For this review, take the finished solid that the model builds, in its own axes (mm). A direction names the side the tool comes from. Round coordinates to 2 decimals unless told otherwise and drop trailing zeros. Write each loop counter-clockwise with the first axis right and the second up, starting at its lowest first coordinate (ties: lowest second). Pieces come first, ordered by that corner, then holes. Notation, with made-up numbers: (42.5, 15.25) -> (51.5, 15.25) arc R25 ccw to (51.5, 35.25) -> close; hole circle Ø11 at (57, -23). An arc over 180 degrees is marked (long way). Answer in a Markdown table with one row per item. Add a question column.
Solid Edge part; units mm, degrees
sketch "Sketch1" plane through (0, 0, 0) normal (0, 0, 1) x (1, 0, 0)
  line L0 (-28.9647, 0) -> (-28.9647, 39.8)
  line L1 (-28.9647, 39.8) -> (-11.9647, 39.8)
  arc A0 (-11.9647, 39.8) -> (-8.8647, 38.9694) centre (-11.9647, 33.6) cw
  line L2 (14.8644, 25.2694) -> (-8.8647, 38.9694)
  arc A1 (14.8644, 14.5306) -> (14.8644, 25.2694) centre (11.7644, 19.9) ccw
  line L3 (-8.8647, 0.8306) -> (14.8644, 14.5306)
  arc A2 (-11.9647, 0) -> (-8.8647, 0.8306) centre (-11.9647, 6.2) ccw
  line L4 (-28.9647, 0) -> (-11.9647, 0)
extrude "Protrusion1" add sketch "Sketch1" along normal blind 10
sketch "Sketch2" plane through (-5.5002, 19.9, 10) normal (0, 0, 1) x (1, 0, 0)
  circle A0 centre (1.4355, 0.0168) radius 2.65
extrude "ExtrudedCutout_1" cut sketch "Sketch2" against normal blind 233.7228
sketch "Sketch3" plane through (-5.5002, 19.9, 0) normal (0, 0, -1) x (1, 0, 0)
  line L0 (-3.6741, -2.9668) -> (-3.6741, 2.9332)
  line L1 (-3.6741, 2.9332) -> (1.4355, 5.8832)
  line L2 (1.4355, 5.8832) -> (6.545, 2.9332)
  line L3 (6.545, 2.9332) -> (6.545, -2.9668)
  line L4 (6.545, -2.9668) -> (1.4355, -5.9168)
  line L5 (1.4355, -5.9168) -> (-3.6741, -2.9668)
extrude "ExtrudedCutout_2" cut sketch "Sketch3" against normal blind 4.9
1. The part is to be moulded in two halves that separate along X. For faces 1 (the flat face through (1.045, 20, 2)), 2 (the flat face through (-9.174, 20, 2)), 3 (the cylindrical face through (17.964, 19.991, 4.93)), 4 (the flat face through (-10, 20, 0)), say which applies: pulls with the +X half, pulls with the -X half, needs draft (parallel to the pull), parting line crosses it, or undercut.
2. For L1, parallel to Z at x = -5.5, y = 15; L2, parallel to X at y = 19, z = 9.75; L3, parallel to Y at x = -6.5, z = 5, list the stretches that pass through material, from the lowest coordinate up. Write a range as [from, to].
3. We need section D-D (y = 16). Write out the cut boundary in (x, z), plus the area to 3 significant figures.
4. Tool access review of faces 5 (the flat face through (-28.965, 20, 5)), 6 (the flat face through (-6.655, 15.512, 2.416)): name each direction out of +Z, -Z, +X, -X, +Y, -Y from which nothing blocks a thin tool from reaching the whole face with its end or side.
5. We need section A-A (y = 21). Write out the cut boundary in (x, z), plus the area to 3 significant figures.
6. We need section C-C (x = -0.5). Write out the cut boundary in (y, z), plus the area to 3 significant figures.
7. We need section B-B (z = 2.5). Write out the cut boundary in (x, y), plus the area to 3 significant figures.
8. Clearance check with flat-ended pins moving along their axes: pin 1 Ø2 at (y, z) = (27, 2.5) entering from +X; pin 2 Ø4 at (y, z) = (19.5, 3.5) entering from +X; pin 3 Ø1.5 at (y, z) = (4, 6.5) entering from +X; pin 4 Ø2 at (x, z) = (-2, 6.5) entering from +Y. State where each tip first meets the part, or that it passes through.
Response:
| question | item | result |
|---|---|---|
| 1 | face 1 | undercut |
| 1 | face 2 | undercut |
| 1 | face 3 | pulls with the +X half |
| 1 | face 4 | needs draft |
| 2 | L1 | [4.9, 10] |
| 2 | L2 | [-28.96, -6.55], [-1.58, 17.9] |
| 2 | L3 | [2.2, 18.87], [20.96, 37.6] |
| 3 | outline | (-28.96, 0) -> (-7.5, 0) -> (-7.5, 4.9) -> (-0.63, 4.9) -> (-0.63, 0) -> (16.58, 0) -> (16.58, 10) -> (-28.96, 10) -> close |
| 3 | area | 422 mm2 |
| 4 | face 5 | +Z, -Z, -X, +Y, -Y |
| 4 | face 6 | -Z |
| 5 | outline | (-28.96, 0) -> (-9.17, 0) -> (-9.17, 4.9) -> (-6.48, 4.9) -> (-6.48, 10) -> (-28.96, 10) -> close; (-1.65, 4.9) -> (1.04, 4.9) -> (1.04, 0) -> (17.87, 0) -> (17.87, 10) -> (-1.65, 10) -> close |
| 5 | area | 394 mm2 |
| 6 | outline | (5.66, 0) -> (16.07, 0) -> (16.07, 4.9) -> (23.76, 4.9) -> (23.76, 0) -> (34.14, 0) -> (34.14, 10) -> (5.66, 10) -> close |
| 6 | area | 247 mm2 |
| 7 | outline | (-28.96, 0) -> (-11.96, 0) arc R6.2 ccw to (-8.86, 0.83) -> (14.86, 14.53) arc R6.2 ccw to (14.86, 25.27) -> (-8.86, 38.97) arc R6.2 ccw to (-11.96, 39.8) -> (-28.96, 39.8) -> close; hole (-9.17, 16.97) -> (-4.06, 14.02) -> (1.04, 16.97) -> (1.04, 22.87) -> (-4.06, 25.82) -> (-9.17, 22.87) -> close |
| 7 | area | 1,310 mm2 |
| 8 | pin 1 | x = 13.6 |
| 8 | pin 2 | x = 17.96 |
| 8 | pin 3 | x = -2.08 |
| 8 | pin 4 | y = 35.58 |
